Read the model definition and answer for the solid it produces. Units are mm, in the model's axes. Round coordinates to 2 decimals unless told otherwise and drop trailing zeros. Write each loop counter-clockwise with the first axis right and the second up, starting at its lowest first coordinate (ties: lowest second). Pieces come first, ordered by that corner, then holes. Notation, with made-up numbers: (24, -33) -> (61, -33) arc R20 cw to (61, -5) -> close; hole circle Ø11 at (89, -20). An arc over 180 degrees is marked (long way). Return JSON: item names as keys, results as strings.
from build123d import *

# Parameters (mm, degrees)
CROQUIS1_W              = 42
CROQUIS1_H              = 85
CROQUIS1_R              = 2.05
CROQUIS1_R_2            = 2.55
SALIENTE_EXTRUIR1_DEPTH = 4
CROQUIS5_R              = 11.5
CROQUIS5_R_2            = 1.575
CORTAR_EXTRUIR2_DEPTH   = 5
CHAFL_N1_SIZE           = 4.1


with BuildPart() as part:
    # Croquis1 → Saliente-Extruir1 (new body)
    with BuildSketch(Plane.XY):
        with Locations((21, 42.5)):
            Rectangle(CROQUIS1_W, CROQUIS1_H)
        with Locations((11, 76.8)):
            Circle(CROQUIS1_R, mode=Mode.SUBTRACT)
        with Locations((31, 76.8)):
            Circle(CROQUIS1_R, mode=Mode.SUBTRACT)
        with Locations((31, 56.8)):
            Circle(CROQUIS1_R, mode=Mode.SUBTRACT)
        with Locations((11, 56.8)):
            Circle(CROQUIS1_R, mode=Mode.SUBTRACT)
        with Locations((21, 21.08)):
            Circle(CROQUIS1_R_2, mode=Mode.SUBTRACT)
    extrude(amount=SALIENTE_EXTRUIR1_DEPTH)

    # Croquis5 → Cortar-Extruir2 (cut, through all)
    with BuildSketch(Plane.XY.offset(4)):
        with Locations((21, 21.08)):
            Circle(CROQUIS5_R)
        with Locations((5.5, 36.58)):
            Circle(CROQUIS5_R_2)
        with Locations((36.5, 36.58)):
            Circle(CROQUIS5_R_2)
        with Locations((36.5, 5.58)):
            Circle(CROQUIS5_R_2)
        with Locations((5.5, 5.58)):
            Circle(CROQUIS5_R_2)
    extrude(amount=-CORTAR_EXTRUIR2_DEPTH, mode=Mode.SUBTRACT)

    # Chaflán1
    chafl_n1_edges = [part.edges().sort_by_distance(p)[0] for p in [
        (42, 0, 2),
        (0, 0, 2),
    ]]
    chamfer(chafl_n1_edges, length=CHAFL_N1_SIZE)


solid = part.part
Item 1: Section B-B (y = 76.8) is taken. Give the vertices of the cut face in (x, z), then the cut area to 3 significant figures.
Worked answers:
{"outline": "(0, 0) -> (8.95, 0) -> (8.95, 4) -> (0, 4) -> close; (13.05, 0) -> (28.95, 0) -> (28.95, 4) -> (13.05, 4) -> close; (33.05, 0) -> (42, 0) -> (42, 4) -> (33.05, 4) -> close", "area": "135 mm2"}
Item 2: Straight lines are drawn through the part: L1, parallel to Y at x = 36.5, z = 1.55 (3 decimals); L2, parallel to X at y = 57, z = 1.6; L3, parallel to Y at x = 11, z = 2.05. For each, find the intervals that lie inside material, in ascending order. Write a range as [from, to].
Worked answers:
{"L1": "y = [0, 4.005], [7.155, 35.005], [38.155, 85]", "L2": "x = [0, 8.96], [13.04, 28.96], [33.04, 42]", "L3": "y = [0, 15.4], [26.76, 54.75], [58.85, 74.75], [78.85, 85]"}
Item 3: For a pull along X with two mould halves and no side action, classify faces 1 (the flat face through (21, 0, 2)), 2 (the flat face through (0, 44, 2)), 3 (the cylindrical face through (30.556, 54.799, 1.972)) as released by +X, released by -X, zero draft, split by the parting line, or undercut.
Worked answers:
{"face 1": "zero draft", "face 2": "released by -X", "face 3": "undercut"}
Item 4: Section C-C (z = 1) is taken. State how many separate pieces and enclosed holes the cut face has, then the cut area to 3 significant figures.
Worked answers:
{"separate pieces": "1", "enclosed holes": "9", "area": "3,050 mm2"}
Item 5: Section A-A (x = 36.5) is taken. Give the vertices of the cut face in (y, z) (3 decimals), then the cut area to 3 significant figures.
Worked answers:
{"outline": "(0, 0) -> (4.005, 0) -> (4.005, 4) -> (0, 4) -> close; (7.155, 0) -> (35.005, 0) -> (35.005, 4) -> (7.155, 4) -> close; (38.155, 0) -> (85, 0) -> (85, 4) -> (38.155, 4) -> close", "area": "315 mm2"}
Item 6: A flat-ended cylindrical pin translates along its axis: pin 1 (2 mm diameter, centred on x = 10, y = 57, fed in from +Z). Find the tip coordinate at first contact, or state that the pin passes through.
Worked answers:
{"pin 1": "passes through"}
Item 7: Section D-D (y = 21.08) is taken. Give the vertices of the cut face in (x, z), then the cut area to 3 significant figures.
Worked answers:
{"outline": "(0, 0) -> (9.5, 0) -> (9.5, 4) -> (0, 4) -> close; (32.5, 0) -> (42, 0) -> (42, 4) -> (32.5, 4) -> close", "area": "76.0 mm2"}
